Check sheet for the modelled part. Datum: model origin and axes. Units: mm. A direction names the side the tool comes from. Round coordinates to 2 decimals unless told otherwise and drop trailing zeros. Loops run counter-clockwise (first coordinate to the right, second up) from the corner with the lowest first, then second, coordinate; pieces in that order, holes last. Notation, with made-up numbers: (-24.75, -23) - (11.25, -23) arc R34 ccw to (11.25, 11) - close; hole circle Ø9 at (31.25, 65.5). An arc over 180 degrees is marked (long way). Put each result on its own line as item: value.
```python
from build123d import *

# Parameters (mm, degrees)
CROQUIS1_W              = 184.15
CROQUIS1_H              = 139.7
SALIENTE_EXTRUIR1_DEPTH = 3.1242
CROQUIS2_R              = 1.3335
CORTAR_EXTRUIR1_DEPTH   = 116.613964341
CROQUIS9_R              = 1.27
CORTAR_EXTRUIR6_DEPTH   = 116.613964341
CORTAR_EXTRUIR2_DEPTH   = 116.613964341
CROQUIS5_R              = 1.651
DRIVER_DEPTH            = 116.613964341
CROQUIS6_R              = 1.651
RASPI_DEPTH             = 116.613964341
CROQUIS8_R              = 1.27
CORTAR_EXTRUIR5_DEPTH   = 116.613964341
CROQUIS7_W              = 11.1125
CROQUIS7_H              = 2.9972
CORTAR_EXTRUIR7_DEPTH   = 116.613964341


with BuildPart() as part:
    # Croquis1 → Saliente-Extruir1 (new body)
    with BuildSketch(Plane.XY):
        Rectangle(CROQUIS1_W, CROQUIS1_H)
    extrude(amount=SALIENTE_EXTRUIR1_DEPTH)

    # Croquis2 → Cortar-Extruir1 (cut, through all)
    with BuildSketch(Plane.XY.offset(3.1242)):
        with BuildLine():
            ThreePointArc((68.2879, 61.5442), (67.636840382, 62.689842778), (66.3194, 62.716802767))
            Line((66.3194, 62.716802767), (66.3194, 60.371597233))
            ThreePointArc((66.3194, 60.371597233), (67.636840382, 60.398557222), (68.2879, 61.5442))
        make_face()
        with BuildLine():
            Line((66.3194, 60.371597233), (66.3194, 62.716802767))
            ThreePointArc((66.3194, 62.716802767), (65.6209, 61.5442), (66.3194, 60.371597233))
        make_face()
        with Locations(Location((66.9544, -61.5442, 0), (0, 0, 180))):
            Circle(CROQUIS2_R)
    extrude(amount=-CORTAR_EXTRUIR1_DEPTH, mode=Mode.SUBTRACT)

    # Croquis9 → Cortar-Extruir6 (cut, through all)
    with BuildSketch(Plane.XY.offset(3.1242)):
        with Locations((52.2859, 38.4937)):
            Circle(CROQUIS9_R)
        with Locations((81.6229, 38.4937)):
            Circle(CROQUIS9_R)
        with Locations(Location((81.6229, -38.4937, 0), (0, 0, 180))):
            Circle(CROQUIS9_R)
        with Locations(Location((52.2859, -38.4937, 0), (0, 0, 180))):
            Circle(CROQUIS9_R)
    extrude(amount=-CORTAR_EXTRUIR6_DEPTH, mode=Mode.SUBTRACT)

    # Croquis3 → Cortar-Extruir2 (cut, through all)
    with BuildSketch(Plane.XY.offset(3.1242)):
        with BuildLine():
            ThreePointArc((19.05, 69.85), (23.540128061, 67.990128061), (25.4, 63.5))
            Line((25.4, 63.5), (25.4, 62.214355717))
            ThreePointArc((25.4, 62.214355717), (31.009401302, 49.616015934), (43.79595, 44.45))
            Line((43.79595, 44.45), (46.307334449, 44.45))
            ThreePointArc((46.307334449, 44.45), (57.607742834, 49.876604957), (62.1919, 61.5442))
            ThreePointArc((62.1919, 61.5442), (65.45872604, 66.06574461), (70.77746038, 64.384202742))
            ThreePointArc((70.77746038, 64.384202742), (86.61242756, 33.907634674), (92.075, 0))
            Line((92.075, 0), (92.075, 69.85))
            Line((92.075, 69.85), (19.05, 69.85))
        make_face()
        with BuildLine():
            Line((92.075, -69.85), (92.075, 0))
            ThreePointArc((92.075, 0), (86.61242756, -33.907634674), (70.77746038, -64.384202742))
            ThreePointArc((70.77746038, -64.384202742), (65.45872604, -66.06574461), (62.1919, -61.5442))
            ThreePointArc((62.1919, -61.5442), (57.607742834, -49.876604957), (46.307334449, -44.45))
            Line((46.307334449, -44.45), (43.79595, -44.45))
            ThreePointArc((43.79595, -44.45), (31.009401302, -49.616015934), (25.4, -62.214355717))
            Line((25.4, -62.214355717), (25.4, -63.5))
            ThreePointArc((25.4, -63.5), (23.540128061, -67.990128061), (19.05, -69.85))
            Line((19.05, -69.85), (92.075, -69.85))
        make_face()
        with BuildLine():
            ThreePointArc((-92.075, 60.325), (-89.285192091, 67.060192091), (-82.55, 69.85))
            Line((-82.55, 69.85), (-92.075, 69.85))
            Line((-92.075, 69.85), (-92.075, 60.325))
        make_face()
        with BuildLine():
            Line((-92.075, -69.85), (-82.55, -69.85))
            ThreePointArc((-82.55, -69.85), (-89.285192091, -67.060192091), (-92.075, -60.325))
            Line((-92.075, -60.325), (-92.075, -69.85))
        make_face()
    extrude(amount=-CORTAR_EXTRUIR2_DEPTH, mode=Mode.SUBTRACT)

    # Croquis5 → Driver (cut, through all)
    with BuildSketch(Plane.XY.offset(3.1242)):
        with BuildLine():
            Line((12.47775, -16.1036), (-18.82775, -16.1036))
            ThreePointArc((-18.82775, -16.1036), (-19.389016008, -16.336083992), (-19.6215, -16.89735))
            Line((-19.6215, -16.89735), (-19.6215, -22.7076))
            ThreePointArc((-19.6215, -22.7076), (-20.55143597, -24.95266403), (-22.7965, -25.8826))
            Line((-22.7965, -25.8826), (-24.7015, -25.8826))
            ThreePointArc((-24.7015, -25.8826), (-28.293602448, -27.370497552), (-29.7815, -30.9626))
            Line((-29.7815, -30.9626), (-29.7815, -51.816))
            ThreePointArc((-29.7815, -51.816), (-28.293602448, -55.408102448), (-24.7015, -56.896))
            Line((-24.7015, -56.896), (-22.7965, -56.896))
            ThreePointArc((-22.7965, -56.896), (-20.55143597, -57.82593597), (-19.6215, -60.071))
            Line((-19.6215, -60.071), (-19.6215, -65.88125))
            ThreePointArc((-19.6215, -65.88125), (-19.389016008, -66.442516008), (-18.82775, -66.675))
            Line((-18.82775, -66.675), (12.47775, -66.675))
            ThreePointArc((12.47775, -66.675), (13.039016008, -66.442516008), (13.2715, -65.88125))
            Line((13.2715, -65.88125), (13.2715, -56.388))
            ThreePointArc((13.2715, -56.388), (14.350225725, -53.783725725), (16.9545, -52.705))
            Line((16.9545, -52.705), (19.05, -52.705))
            ThreePointArc((19.05, -52.705), (20.172532015, -52.240032015), (20.6375, -51.1175))
            Line((20.6375, -51.1175), (20.6375, -31.6611))
            ThreePointArc((20.6375, -31.6611), (20.172532015, -30.538567985), (19.05, -30.0736))
            Line((19.05, -30.0736), (16.9545, -30.0736))
            ThreePointArc((16.9545, -30.0736), (14.350225725, -28.994874275), (13.2715, -26.3906))
            Line((13.2715, -26.3906), (13.2715, -16.89735))
            ThreePointArc((13.2715, -16.89735), (13.039016008, -16.336083992), (12.47775, -16.1036))
        make_face()
        with Locations((17.0815, -21.5646)):
            Circle(CROQUIS5_R)
        with Locations((-23.0505, -21.4376)):
            Circle(CROQUIS5_R)
        with Locations(Location((17.0815, -61.214, 0), (0, 0, 180))):
            Circle(CROQUIS5_R)
        with Locations(Location((-23.0505, -61.341, 0), (0, 0, 180))):
            Circle(CROQUIS5_R)
    extrude(amount=-DRIVER_DEPTH, mode=Mode.SUBTRACT)

    # Croquis6 → RasPi (cut, through all)
    with BuildSketch(Plane.XY.offset(3.1242)):
        with Locations((-29.95, 48.2464)):
            Circle(CROQUIS6_R)
        with Locations((19.05, 48.2464)):
            Circle(CROQUIS6_R)
        with Locations((19.05, -9.7536)):
            Circle(CROQUIS6_R)
        with Locations((-29.95, -9.7536)):
            Circle(CROQUIS6_R)
    extrude(amount=-RASPI_DEPTH, mode=Mode.SUBTRACT)

    # Croquis8 → Cortar-Extruir5 (cut, through all)
    with BuildSketch(Plane.XY.offset(3.1242)):
        with Locations((-83.185, 61.138037406)):
            Circle(CROQUIS8_R)
        with Locations((-55.795218831, 33.748256237)):
            Circle(CROQUIS8_R)
    extrude(amount=-CORTAR_EXTRUIR5_DEPTH, mode=Mode.SUBTRACT)

    # Croquis7 → Cortar-Extruir7 (cut, through all)
    with BuildSketch(Plane.XY.offset(3.1242)):
        with Locations((-69.490109415, -63.5889)):
            Rectangle(CROQUIS7_W, CROQUIS7_H)
    extrude(amount=-CORTAR_EXTRUIR7_DEPTH, mode=Mode.SUBTRACT)


solid = part.part
```
Item 1: Tool access check on faces 1 (the flat face through (-1, 1, 0)), 2 (the cylindrical face through (57.485, 49.746, 1.584)), 3 (the cylindrical face through (-28.3, -55.4, 1.6)), 4 (the cylindrical face through (23.59, -67.94, 1.58)). Record the directions out of +Z, -Z, +X, -X, +Y, -Y that give a thin tool (end or side, any length) a straight path to the whole face; none if there is none.
Filled sheet:
face 1: -Z, +X, -X, +Y, -Y
face 2: +Z, -Z, +Y
face 3: +Z, -Z
face 4: +Z, -Z, -Y
Item 2: Go/stop test with flat-tipped pins: pin 1 (0.6 mm diameter, centred on y = 62.5, z = 1, fed in from +X); pin 2 (1.6 mm diameter, centred on y = -38.5, z = 2.5, fed in from +X); pin 3 (0.9 mm diameter, centred on y = -63.5, z = 2, fed in from +X). Record where each tip stops, or that it passes through.
Filled sheet:
pin 1: x = 72.36
pin 2: x = 85.28
pin 3: x = 71.75
Item 3: Release check for a two-part mould opening along Y. For faces 5 (the cylindrical face through (-89.359, 66.986, 1.584)), 6 (the cylindrical face through (57.73, -50.01, 1.58)), 7 (the cylindrical face through (14.379, -29.023, 1.584)), 8 (the cylindrical face through (-28.25, -27.33, 1.58)) record: +Y half, -Y half, draft (parallel to the pull), parting line (faces both ways), or undercut.
Filled sheet:
face 5: +Y half
face 6: -Y half
face 7: undercut
face 8: undercut
Item 4: Section check A-A on x = -72. Enter the section's corners in (y, z).
Filled sheet:
outline: (-69.85, 0) - (-65.09, 0) - (-65.09, 3.12) - (-69.85, 3.12) - close; (-62.09, 0) - (69.85, 0) - (69.85, 3.12) - (-62.09, 3.12) - close
Item 5: Section check B-B on z = 1.65. Count the separate pieces of the cut face and the enclosed holes in it, then the cut area to 3 significant figures.
Filled sheet:
separate pieces: 1
enclosed holes: 18
area: 20,600 mm²
Item 6: Thickness scan on line 1 (Y direction, x = -30, z = 0.9); line 2 (X direction, y = -52.5, z = 0.3) (3 decimals); line 3 (Y direction, x = 6.5, z = 0.35) (3 decimals). Record the ranges inside material, lowest first. Write a range as from..to.
Filled sheet:
line 1: -69.85..-11.4, -8.1..46.6, 49.9..69.85
line 2: -92.075..-29.735, 19.83..28.579, 59.612..78.451
line 3: -69.85..-66.675, -16.104..69.85
